from build123d import *

# Parameters (mm, degrees)
F1_DEPTH        = 30
F2_W            = 30
F2_H            = 38
F2_W_2          = 7.5
F2_H_2          = 20
F2_W_3          = 20
F2_H_3          = 5
F3_DEPTH        = 42
F4_R            = 4.75
F4_R_2          = 2.75
F5_DEPTH        = 22
F6_DEPTH        = 42
F8_D            = 8
F8_DEPTH        = 9
F8_TIP          = 2.4034424761
F10_D           = 8
F10_DEPTH       = 50
F10_CBORE_D     = 10
F10_CBORE_DEPTH = 2
F10_TIP         = 2.4034424761
F11_D           = 8
F11_DEPTH       = 50
F11_TIP         = 2.4034424761


with BuildPart() as f1:
    # F0 (on Right) → F1 (new body, symmetric)
    with BuildSketch(Plane.YZ):
        Polygon((21, -40), (21, 40), (1, 40), (-21, 8), (-21, -40), align=None)
    extrude(amount=F1_DEPTH, both=True)

    # F2 (on face) → F3 (cut)
    with BuildSketch(Plane.XZ.offset(21)):
        Polygon((30, 8), (30, 40), (25, 40), (25, 5), (30, -10), align=None)
        with Locations((0, 21)):
            Rectangle(F2_W, F2_H)
        with Locations((-26.25, -30)):
            Rectangle(F2_W_2, F2_H_2)
        with Locations((26.25, -30)):
            Rectangle(F2_W_2, F2_H_2)
        Polygon((-30, -10), (-25, 5), (-25, 40), (-30, 40), (-30, 8), align=None)
        with Locations((0, -37.5)):
            Rectangle(F2_W_3, F2_H_3)
    extrude(amount=-F3_DEPTH, mode=Mode.SUBTRACT)

    # F4 (on face) → F5 (cut)
    with BuildSketch(Plane.XZ.offset(21)):
        with Locations((15, -29)):
            Circle(F4_R)
        with Locations((15, -29)):
            Circle(F4_R_2, mode=Mode.SUBTRACT)
        with Locations((-15, -29)):
            Circle(F4_R)
        with Locations((-15, -29)):
            Circle(F4_R_2, mode=Mode.SUBTRACT)
        with Locations((-15, -29)):
            Circle(F4_R_2)
        with Locations((15, -29)):
            Circle(F4_R_2)
    extrude(amount=-F5_DEPTH, mode=Mode.SUBTRACT)

    # F4 (on face) → F6 (cut)
    with BuildSketch(Plane.XZ.offset(21)):
        with Locations((-15, -29)):
            Circle(F4_R_2)
        with Locations((15, -29)):
            Circle(F4_R_2)
    extrude(amount=-F6_DEPTH, mode=Mode.SUBTRACT)

    # F8
    with Locations(Plane.XY.offset(2)):
        with Locations((0, 11)):
            Hole(F8_D / 2, depth=F8_DEPTH)
            with Locations((0, 0, -(F8_DEPTH + F8_TIP / 2))):  # 118° drill point
                Cone(0, F8_D / 2, F8_TIP, mode=Mode.SUBTRACT)

    # F10
    with Locations(Plane(origin=(-25, 0, 0), x_dir=(0, -1, 0), z_dir=(-1, 0, 0))):
        with Locations((-13, 32)):
            CounterBoreHole(F10_D / 2, F10_CBORE_D / 2, F10_CBORE_DEPTH, depth=F10_DEPTH)
            with Locations((0, 0, -(F10_DEPTH + F10_TIP / 2))):  # 118° drill point
                Cone(0, F10_D / 2, F10_TIP, mode=Mode.SUBTRACT)

    # F11
    with Locations(Plane(origin=(-25, 0, 0), x_dir=(0, -1, 0), z_dir=(-1, 0, 0))):
        with Locations((9, 14)):
            Hole(F11_D / 2, depth=F11_DEPTH)
            with Locations((0, 0, -(F11_DEPTH + F11_TIP / 2))):  # 118° drill point
                Cone(0, F11_D / 2, F11_TIP, mode=Mode.SUBTRACT)


solid = f1.part
Work out the finished part from the listing and answer in its coordinate system (mm). A direction names the side the tool comes from. Give positions to 0.01 mm unless a question says otherwise; leave off trailing zeros. Order: outer loops, then holes, each group sorted by start corner. A loop starts at its lowest first (then second) coordinate and runs counter-clockwise, first axis right, second up. Notation, with made-up numbers: (54, -26) -> (74, -26) arc R5 ccw to (74, -18) -> close; hole circle Ø7 at (4, 89). An arc over 180 degrees is marked (long way). Answer as a JSON object with one key per item and string values. Group by question number.
1. The mould has two halves that part along Z. Classify faces 1 (the flat face through (-15, 1, -32)), 2 (the flat face through (15, 4, 17)), 3 (the flat face through (20, -10, 24)), 4 (the cylindrical face through (-18.944, 12.479, 35.966)): released by +Z, released by -Z, zero draft, split by the parting line, or undercut.
2. Flat-ended cylindrical pins translate along their axes: pin 1 Ø5.5 at (y, z) = (2, -36.5) entering from -X; pin 2 Ø1.5 at (y, z) = (9.5, 7) entering from -X; pin 3 Ø17.5 at (y, z) = (-1.5, 21.5) entering from +X. Find the tip coordinate at first contact, or state that the pin passes through.
3. A tool of negligible diameter and unlimited length cuts with its end or side. For faces 5 (the cylindrical face through (0.521, 14.966, -2.563)), 6 (the cylindrical face through (-16.03, -10.154, -33.637)), 7 (the flat face through (0, 0, -35)), from which of +Z, -Z, +X, -X, +Y, -Y can it reach the whole face along a straight path? Write none if from no direction.
4. Consider line 1 along X through (y, z) = (-6, 29); line 2 along X through (y, z) = (-2, -21.5); line 3 along Z through (x, y) = (23.5, 13). Determine where each line is inside the solid, lowest interval first. Write a range as [from, to].
5. Section B-B on y = -9 is taken. Count the separate pieces of the cut face and the enclosed holes in it, plus the area to 3 significant figures.
6. Section D-D on x = -8 is taken. Determine the outline of the cut face in (y, z), plus the area to 3 significant figures.
7. Section A-A on z = 32 is taken. Determine the outline of the cut face in (x, y).
8. Section C-C on y = 3.5 is taken. Determine the outline of the cut face in (x, z).
Result sheet:
{
 "1": {"face 1": "undercut", "face 2": "zero draft", "face 3": "released by +Z", "face 4": "undercut"},
 "2": {"pin 1": "stops at x = -22.5", "pin 2": "stops at x = -25", "pin 3": "stops at x = 25"},
 "3": {"face 5": "+Z", "face 6": "-Y", "face 7": "-Z, +Y, -Y"},
 "4": {"line 1": "x = [-25, -15], [15, 25]", "line 2": "x = [-22.5, 22.5]", "line 3": "z = [-20, 28], [36, 40]"},
 "5": {"separate pieces": "3", "enclosed holes": "2", "area": "2,240 mm^2"},
 "6": {"outline": "(-21, -35) -> (21, -35) -> (21, 2) -> (-21, 2) -> close", "area": "1,550 mm^2"},
 "7": {"outline": "(-25, -4.5) -> (-15, -4.5) -> (-15, 9) -> (-23, 9) -> (-23, 8) -> (-25, 8) -> close; (-25, 18) -> (-23, 18) -> (-23, 17) -> (-15, 17) -> (-15, 21) -> (-25, 21) -> close; (15, -4.5) -> (25, -4.5) -> (25, 9) -> (15, 9) -> close; (15, 17) -> (25, 17) -> (25, 21) -> (15, 21) -> close"},
 "8": {"outline": "(-30, -20) -> (-22.5, -20) -> (-22.5, -40) -> (-10, -40) -> (-10, -35) -> (10, -35) -> (10, -40) -> (22.5, -40) -> (22.5, -20) -> (30, -20) -> (30, -10) -> (25, 5) -> (25, 40) -> (15, 40) -> (15, 2) -> (-15, 2) -> (-15, 40) -> (-25, 40) -> (-25, 5) -> (-30, -10) -> close; hole circle Ø5.5 at (-15, -29); hole circle Ø5.5 at (15, -29)"}
}
